from build123d import *

# Parameters (mm, degrees)
SKETCH_W    = 70
SKETCH_H    = 70
PAD_DEPTH   = 20
SKETCH002_W = 20
SKETCH002_H = 20
SKETCH001_W = 30
SKETCH001_H = 30
FILLET_R    = 2


with BuildPart() as part:
    # Sketch → Pad (new body)
    with BuildSketch(Plane.XY):
        with Locations((-35, -35)):
            Rectangle(SKETCH_W, SKETCH_H)
    extrude(amount=PAD_DEPTH)

    # Sketch002 (on DatumPlane) → SubtractiveLoft section 0
    with BuildSketch(Plane.XY.offset(10)):
        with Locations((-35, -35)):
            Rectangle(SKETCH002_W, SKETCH002_H)
    # Sketch001 (on Face6 of Pad) → SubtractiveLoft section 1
    with BuildSketch(Plane.XY.offset(20)):
        with Locations((-35, -35)):
            Rectangle(SKETCH001_W, SKETCH001_H)
    loft(mode=Mode.SUBTRACT)

    # Fillet
    fillet_edges = [part.edges().sort_by_distance(p)[0] for p in [
        (-45, -35, 10),
        (-47.5, -47.5, 15),
        (-50, -35, 20),
        (-47.5, -22.5, 15),
        (-35, -25, 10),
        (-35, -20, 20),
        (-22.5, -22.5, 15),
        (-25, -35, 10),
        (-20, -35, 20),
        (-22.5, -47.5, 15),
        (-35, -45, 10),
        (-35, -50, 20),
    ]]
    fillet(fillet_edges, radius=FILLET_R)


solid = part.part
CAD build for the part. Positions are in the model's coordinates, mm. Give positions to 0.01 mm unless a question says otherwise; leave off trailing zeros. Write each question's results on one line, items separated by ' | '.
1. Pin check, flat tip, straight feed: pin 1 (5.5 mm diameter, centred on x = -36.5, y = -36, fed in from +Z). Stop position of the tip, or through.
Calculated:
pin 1: stops at z = 10
2. Pull direction Y, two halves, no side cores. Call faces 1 (the face through (-35, 0, 10)), 2 (the face through (-51, -19, 20)), 3 (the face through (-35, -35, 10)): released by +Y, released by -Y, zero draft, split by the parting line, or undercut.
Calculated:
face 1: released by +Y | face 2: zero draft | face 3: undercut
3. Probe L1, parallel to X at y = -26.5, z = 11.25 (3 decimals); L2, parallel to Z at x = -36, y = -29; L3, parallel to X at y = -47, z = 18.5. List the from-to ranges inside material, lowest first. Write a range as from..to.
Calculated:
L1: x = -70..-45.625, -24.375..0 | L2: z = 0..10 | L3: x = -70..-49.25, -20.75..0
